```python
from build123d import *

# Parameters (mm, degrees)
SKETCH1_R           = 2.5
BOSS_EXTRUDE2_DEPTH = 2
FLEX1_OUTLINE_R     = 2.5
FLEX1_DEPTH         = 2


# Read off the part's stored shape, not the designer's step: Flex1
with BuildPart() as part:
    # Sketch1 → Boss-Extrude2 (new body)
    with BuildSketch(Plane(origin=(0, 0, 0), x_dir=(1, 0, 0), z_dir=(0, 1, 0))):
        with BuildLine():
            Line((2.5, 0), (47.5, 0))
            ThreePointArc((47.5, 0), (49.267766953, 0.732233047), (50, 2.5))
            Line((50, 2.5), (50, 7.5))
            ThreePointArc((50, 7.5), (49.267766953, 9.267766953), (47.5, 10))
            Line((47.5, 10), (2.5, 10))
            ThreePointArc((2.5, 10), (0.732233047, 9.267766953), (0, 7.5))
            Line((0, 7.5), (0, 2.5))
            ThreePointArc((0, 2.5), (0.732233047, 0.732233047), (2.5, 0))
        make_face()
        with Locations(Location((5, 5, 0), (0, 0, 270))):
            Circle(SKETCH1_R, mode=Mode.SUBTRACT)
        with Locations(Location((45, 5, 0), (0, 0, 270))):
            Circle(SKETCH1_R, mode=Mode.SUBTRACT)
    extrude(amount=BOSS_EXTRUDE2_DEPTH)

    # Flex1 outline → Flex1 (add)
    # profile 1 of 4: a face of its own
    with BuildSketch(Plane(origin=(0, 0, 0), x_dir=(1, 0, 0), z_dir=(0, 1, 0))):
        with BuildLine():
            Line((2.5, 10), (-158.5152852, 10))
            ThreePointArc((-158.5152852, 10), (-160.283052153, 9.267766953), (-161.0152852, 7.5))
            Line((-161.0152852, 7.5), (-161.0152852, 2.5))
            ThreePointArc((-161.0152852, 2.5), (-160.283052153, 0.732233047), (-158.5152852, 0))
            Line((-158.5152852, 0), (2.5, 0))
            ThreePointArc((2.5, 0), (0.732233047, 0.732233047), (0, 2.5))
            Line((0, 2.5), (0, 7.5))
            ThreePointArc((0, 7.5), (0.732233047, 9.267766953), (2.5, 10))
        make_face()
        with Locations((-156.0152852, 5)):
            Circle(FLEX1_OUTLINE_R, mode=Mode.SUBTRACT)
    # profile 2 of 4: a face of its own
    with BuildSketch(Plane(origin=(0, 0, 0), x_dir=(1, 0, 0), z_dir=(0, 1, 0))):
        with BuildLine():
            Line((216.4847148, 10), (47.5, 10))
            ThreePointArc((47.5, 10), (49.267766953, 9.267766953), (50, 7.5))
            Line((50, 7.5), (50, 2.5))
            ThreePointArc((50, 2.5), (49.267766953, 0.732233047), (47.5, 0))
            Line((47.5, 0), (216.4847148, 0))
            ThreePointArc((216.4847148, 0), (218.252481753, 0.732233047), (218.9847148, 2.5))
            Line((218.9847148, 2.5), (218.9847148, 7.5))
            ThreePointArc((218.9847148, 7.5), (218.252481753, 9.267766953), (216.4847148, 10))
        make_face()
        with Locations((213.9847148, 5)):
            Circle(FLEX1_OUTLINE_R, mode=Mode.SUBTRACT)
    # profile 3 of 4: a face of its own
    with BuildSketch(Plane(origin=(0, 0, 0), x_dir=(1, 0, 0), z_dir=(0, 1, 0))):
        with Locations((5, 5)):
            Circle(FLEX1_OUTLINE_R)
    # profile 4 of 4: a face of its own
    with BuildSketch(Plane(origin=(0, 0, 0), x_dir=(1, 0, 0), z_dir=(0, 1, 0))):
        with Locations((45, 5)):
            Circle(FLEX1_OUTLINE_R)
    extrude(amount=FLEX1_DEPTH)


solid = part.part
```
Input: part model. Units: mm. Frame: model coordinates. Give positions to 0.01 mm unless a question says otherwise; leave off trailing zeros. Order: outer loops, then holes, each group sorted by start corner. A loop starts at its lowest first (then second) coordinate and runs counter-clockwise, first axis right, second up.
1. Section A-A on z = -5. Return the cut outline in (x, y), and give its area (3 significant figures).
Derived:
outline: (-161.02, 0) - (-158.52, 0) - (-158.52, 2) - (-161.02, 2) - close; (-153.52, 0) - (211.48, 0) - (211.48, 2) - (-153.52, 2) - close; (216.48, 0) - (218.98, 0) - (218.98, 2) - (216.48, 2) - close
area: 740 mm2
2. Material intervals for L1, parallel to X at y = 1.3, z = -4.5; L2, parallel to X at y = 1.45, z = -5; L3, parallel to X at y = 1.4, z = -2, sorted ascending.
Derived:
L1: x = -161.02 to -158.46, -153.57 to 211.54, 216.43 to 218.98
L2: x = -161.02 to -158.52, -153.52 to 211.48, 216.48 to 218.98
L3: x = -160.96 to 218.93
3. Pin query (flat end, axial travel): pin 1 (4.5 mm diameter, centred on x = -156.02, z = -5, fed in from -Y). Return the tip coordinate at first contact, or that it passes through.
Derived:
pin 1: passes through
